Part model, mm, in its own coordinate system. A direction names the side the tool comes from. Round coordinates to 2 decimals unless told otherwise and drop trailing zeros. Loops run counter-clockwise (first coordinate to the right, second up) from the corner with the lowest first, then second, coordinate; pieces in that order, holes last.
1) Mould opens along Y. For faces 1 (the flat face through (124, 179.589, 1)), 2 (the cylindrical face through (138.182, 186.854, 1.479)), 3 (the flat face through (124, 193, 0)) say: +Y half, -Y half, draft (parallel to the pull), parting line (faces both ways), or undercut.
2) Band-saw the part on B-B, the plane z = 0.4. State how many separate pieces and enclosed holes the cut face has, then the cut area to 3 significant figures.
3) 3-axis set-ups, long thin cutter, end or side, ignore diameter. For faces 4 (the flat face through (110.375, 180, 1)), 5 (the flat face through (110, 202.089, 1)), 6 (the flat face through (137.375, 180, 1)), 7 (the flat face through (108, 205.089, 1)): which of +Z, -Z, +X, -X, +Y, -Y reach the whole face in a straight line?
4) Probe line 1 (X direction, y = 194.5, z = 0.5); line 2 (Y direction, x = 110, z = 1.2); line 3 (X direction, y = 193.5, z = 1.35). List the from-to ranges inside material, lowest first.
5) Band-saw the part on D-D, the plane x = 109.5. Write the cut outline in (y, z).
6) Drop flat-ended pins along their axis: P1, Ø2.5, axis at x = 128.38, y = 200.59, coming from the -Z side; P2, Ø1.6, axis at y = 200.5, z = 2, coming from the -X side; P3, Ø0.9, axis at x = 108.5, z = 1, coming from the +Y side. Give the stop position or say it passes through.
7) Band-saw the part on A-A, the plane x = 134. Write the cut outline in (y, z).
8) Band-saw the part on C-C, the plane x = 138. Write the cut outline in (y, z).
from build123d import *

# Parameters (mm, degrees)
MODEL_R                 = 1.5
SALIENTE_EXTRUIR1_DEPTH = 3


with BuildPart() as part:
    # Model → Saliente-Extruir1 (new body)
    with BuildSketch(Plane.XY):
        with BuildLine():
            Line((105.875172656, 202.089330986), (105.875172656, 205.089330986))
            Line((105.875172656, 205.089330986), (110.375172306, 205.089330986))
            Line((110.375172306, 205.089330986), (110.375172306, 206.589330986))
            Line((110.375172306, 206.589330986), (137.375172656, 206.589330986))
            Line((137.375172656, 206.589330986), (137.375172656, 205.089330986))
            Line((137.375172656, 205.089330986), (141.875172656, 205.089330986))
            Line((141.875172656, 205.089330986), (141.875172656, 202.089330986))
            Line((141.875172656, 202.089330986), (133.625172656, 202.089319857))
            ThreePointArc((133.625172656, 202.089319857), (133.094842866, 201.869649228), (132.875173667, 201.339318846))
            Line((132.875173667, 201.339318846), (132.875175691, 199.839318846))
            ThreePointArc((132.875175691, 199.839318846), (133.09484632, 199.308989056), (133.625176703, 199.089319857))
            Line((133.625176703, 199.089319857), (141.875172656, 199.089330986))
            Line((141.875172656, 199.089330986), (141.875172656, 181.089330986))
            Line((141.875172656, 181.089330986), (137.375172656, 181.089330986))
            Line((137.375172656, 181.089330986), (137.375172656, 179.589330986))
            Line((137.375172656, 179.589330986), (110.375172306, 179.589330986))
            Line((110.375172306, 179.589330986), (110.375172306, 181.089330986))
            Line((110.375172306, 181.089330986), (105.875172656, 181.089330986))
            Line((105.875172656, 181.089330986), (105.875172656, 199.089330986))
            Line((105.875172656, 199.089330986), (114.125172656, 199.089330986))
            ThreePointArc((114.125172656, 199.089330986), (114.655502742, 199.3090009), (114.875172656, 199.839330986))
            Line((114.875172656, 199.839330986), (114.875172656, 201.339330986))
            ThreePointArc((114.875172656, 201.339330986), (114.655502742, 201.869661072), (114.125172656, 202.089330986))
            Line((114.125172656, 202.089330986), (105.875172656, 202.089330986))
        make_face()
        with Locations((128.375172656, 200.589330986)):
            Circle(MODEL_R, mode=Mode.SUBTRACT)
        with Locations((119.375172656, 200.589330986)):
            Circle(MODEL_R, mode=Mode.SUBTRACT)
        with Locations((137.375172306, 185.589330986)):
            Circle(MODEL_R, mode=Mode.SUBTRACT)
        with Locations((128.375172306, 185.589330986)):
            Circle(MODEL_R, mode=Mode.SUBTRACT)
        with Locations((110.375172306, 185.589330986)):
            Circle(MODEL_R, mode=Mode.SUBTRACT)
        with Locations((119.375172306, 185.589330986)):
            Circle(MODEL_R, mode=Mode.SUBTRACT)
        with Locations((137.375172306, 194.589330986)):
            Circle(MODEL_R, mode=Mode.SUBTRACT)
        with Locations((128.375172306, 194.589330986)):
            Circle(MODEL_R, mode=Mode.SUBTRACT)
        with Locations((110.375172306, 194.589330986)):
            Circle(MODEL_R, mode=Mode.SUBTRACT)
        with Locations((119.375172306, 194.589330986)):
            Circle(MODEL_R, mode=Mode.SUBTRACT)
    extrude(amount=SALIENTE_EXTRUIR1_DEPTH)


solid = part.part
Reported:
1. face 1: -Y half
1. face 2: undercut
1. face 3: draft
2. separate pieces: 1
2. enclosed holes: 10
2. area: 821 mm2
3. face 4: +Z, -Z, -X, -Y
3. face 5: +Z, -Z, -X
3. face 6: +Z, -Z, +X, -Y
3. face 7: +Z, -Z, -X, +Y
4. line 1: x = 105.88 to 108.88, 111.87 to 117.88, 120.87 to 126.88, 129.87 to 135.88, 138.87 to 141.88
4. line 2: y = 181.09 to 184.14, 187.04 to 193.14, 196.04 to 199.09, 202.09 to 205.09
4. line 3: x = 105.88 to 109.34, 111.41 to 118.34, 120.41 to 127.34, 129.41 to 136.34, 138.41 to 141.88
5. outline: (181.09, 0) - (184.37, 0) - (184.37, 3) - (181.09, 3) - close; (186.81, 0) - (193.37, 0) - (193.37, 3) - (186.81, 3) - close; (195.81, 0) - (199.09, 0) - (199.09, 3) - (195.81, 3) - close; (202.09, 0) - (205.09, 0) - (205.09, 3) - (202.09, 3) - close
6. P1: passes through
6. P2: stops at x = 114.86
6. P3: stops at y = 205.09
7. outline: (179.59, 0) - (199.09, 0) - (199.09, 3) - (179.59, 3) - close; (202.09, 0) - (206.59, 0) - (206.59, 3) - (202.09, 3) - close
8. outline: (181.09, 0) - (184.23, 0) - (184.23, 3) - (181.09, 3) - close; (186.95, 0) - (193.23, 0) - (193.23, 3) - (186.95, 3) - close; (195.95, 0) - (199.09, 0) - (199.09, 3) - (195.95, 3) - close; (202.09, 0) - (205.09, 0) - (205.09, 3) - (202.09, 3) - close
